Design review of the part built by this model. Coordinates are the model's own, in mm. A direction names the side the tool comes from. Coordinates: 2 decimals unless noted, no trailing zeros. Write each loop counter-clockwise with the first axis right and the second up, starting at its lowest first coordinate (ties: lowest second). Pieces come first, ordered by that corner, then holes. Notation, with made-up numbers: (-24, 21.25) - (19, 21.25) arc R25 cw to (19, 55.25) - close; hole circle Ø2 at (-26, 49). An arc over 180 degrees is marked (long way). One line per item, written item: value.
from build123d import *

# Parameters (mm, degrees)
F0_W     = 480
F0_H     = 370
F1_DEPTH = 130
F2_R     = 50
F4_DEPTH = 110


with BuildPart() as f1:
    # F0 (on Top) → F1 (new body)
    with BuildSketch(Plane.XY):
        Rectangle(F0_W, F0_H)
    extrude(amount=F1_DEPTH)

    # F2
    f2_edges = [f1.edges().sort_by_distance(p)[0] for p in [
        (240, -185, 65),
        (-240, -185, 65),
        (240, 185, 65),
        (-240, 185, 65),
    ]]
    fillet(f2_edges, radius=F2_R)

    # F3 (on face) → F4 (cut)
    with BuildSketch(Plane.XY.offset(130)):
        with BuildLine():
            ThreePointArc((230, 130), (216.819805, 161.819805), (185, 175))
            Line((185, 175), (-185, 175))
            ThreePointArc((-185, 175), (-216.819805, 161.819805), (-230, 130))
            Line((-230, 130), (-230, -130))
            ThreePointArc((-230, -130), (-216.819805, -161.819805), (-185, -175))
            Line((-185, -175), (185, -175))
            ThreePointArc((185, -175), (216.819805, -161.819805), (230, -130))
            Line((230, -130), (230, 130))
        make_face()
    extrude(amount=-F4_DEPTH, mode=Mode.SUBTRACT)


solid = f1.part
1. Consider section C-C, the plane x = -202. Write out the cut boundary in (y, z).
Answer block:
outline: (-183.54, 0) - (183.54, 0) - (183.54, 130) - (171.67, 130) - (171.67, 20) - (-171.67, 20) - (-171.67, 130) - (-183.54, 130) - close
2. Insertion check: pin 1 Ø10 at (x, y) = (-175.5, 90.5) entering from -Z; pin 2 Ø2 at (x, y) = (-97.5, 102) entering from +Z. Each pin has a flat end and moves straight along its axis. Give the tip position at first contact, or say it passes through.
Answer block:
pin 1: stops at z = 0
pin 2: stops at z = 20
3. For faces 1 (the face through (-54, -177, 130)), 2 (the face through (3, 175, 76)), list the 3-axis set-ups (+Z, -Z, +X, -X, +Y, -Y) from which the entire face can be reached by the end or side of a thin tool; tool diameter is ignored.
Answer block:
face 1: +Z, +X, -X, +Y, -Y
face 2: +Z
4. Consider section A-A, the plane z = 48. Write out the cut boundary in (x, y), then the cut area to 3 significant figures.
Answer block:
outline: (-240, -135) arc R50 ccw to (-190, -185) - (190, -185) arc R50 ccw to (240, -135) - (240, 135) arc R50 ccw to (190, 185) - (-190, 185) arc R50 ccw to (-240, 135) - close; hole (-230, -130) arc R45 ccw to (-185, -175) - (185, -175) arc R45 ccw to (230, -130) - (230, 130) arc R45 ccw to (185, 175) - (-185, 175) arc R45 ccw to (-230, 130) - close
area: 16,200 mm^2
5. Consider section B-B, the plane y = 36. Write out the cut boundary in (x, z), then the cut area to 3 significant figures.
Answer block:
outline: (-240, 0) - (240, 0) - (240, 130) - (230, 130) - (230, 20) - (-230, 20) - (-230, 130) - (-240, 130) - close
area: 11,800 mm^2
6. Mouldability with a two-part tool opening along X and no side actions: class faces 3 (the face through (-3, -175, 76)), 4 (the face through (225.742, 169.964, 65.91)), 5 (the face through (216.468, -162.168, 75.77)), 6 (the face through (-3, -185, 64)) as released by +X, released by -X, zero draft, split by the parting line, or undercut.
Answer block:
face 3: undercut
face 4: released by +X
face 5: undercut
face 6: zero draft
7. Wall thickness on line 1 along Y through (x, z) = (139, 71.5); line 2 along X through (y, z) = (-44, 42); line 3 along Z through (x, y) = (11, -50.5): over which ranges is each line inside the solid? List them lowest first.
Answer block:
line 1: y = -185 to -175, 175 to 185
line 2: x = -240 to -230, 230 to 240
line 3: z = 0 to 20
